Read the model definition and answer for the solid it produces. Units are mm, in the model's axes. Face numbers are marked on the shaded views. Give positions to 0.01 mm unless a question says otherwise; leave off trailing zeros. One line per item, written item: value. Start each with the question number.
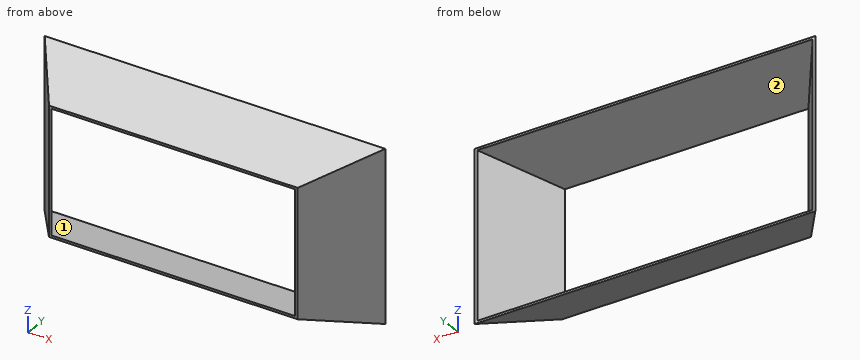
from build123d import *

# Parameters (mm, degrees)
SKETCH2_W = 800
SKETCH2_H = 400
SKETCH1_W = 584
SKETCH1_H = 300
SHELL1_T  = -5


with BuildPart() as part:
    # Sketch2 → Loft1 section 0
    with BuildSketch(Plane(origin=(0, 150, 0), x_dir=(1, 0, 0), z_dir=(0, 1, 0))):
        Rectangle(SKETCH2_W, SKETCH2_H)
    # Sketch1 → Loft1 section 1
    with BuildSketch(Plane(origin=(0, 0, 0), x_dir=(1, 0, 0), z_dir=(0, 1, 0))):
        Rectangle(SKETCH1_W, SKETCH1_H)
    loft()

    # Shell1
    shell1_openings = [part.faces().sort_by_distance(p)[0] for p in [
        (0, 0, 0),
        (0, 150, 0),
    ]]
    offset(amount=SHELL1_T, openings=shell1_openings, kind=Kind.INTERSECTION)


solid = part.part
Item 1: Find the intervals of material crossed by line 1 (X direction, y = 80.5, z = 145); line 2 (X direction, y = 34.5, z = 11.5); line 3 (Z direction, x = -9, y = 11.5), in increasing order. Write a range as from..to.
Item 2: Flat-ended cylindrical pins translate along their axes: pin 1 (4 mm diameter, centred on y = 32, z = 22.5, fed in from +X); pin 2 (2 mm diameter, centred on x = -262, y = 73.5, fed in from -Z); pin 3 (5 mm diameter, centred on x = 165.5, y = 51, fed in from +Z). Find the tip coordinate at first contact, or state that the pin passes through.
Item 3: For a pull along X with two mould halves and no side action, classify the marked faces 1 and 2 as +X half, -X half, draft (parallel to the pull), parting line (faces both ways), or undercut.
Checks:
1. line 1: -349.96..-343.8, 343.8..349.96
1. line 2: -316.84..-310.68, 310.68..316.84
1. line 3: -153.83..-148.56, 148.56..153.83
2. pin 1: x = 316.48
2. pin 2: z = -174.83
2. pin 3: z = 167.83
3. face 1: undercut
3. face 2: undercut
